from build123d import *

# Parameters (mm, degrees)
F0_W     = 76.2
F0_H     = 50.8
F0_R     = 12.7
F1_DEPTH = 12.7
F2_W     = 1.27
F2_H     = 50.8
F3_DEPTH = 5.08
F5_DEPTH = 50.801
F6_R     = 4.7625
F7_DEPTH = 12.7
F8_W     = 12.7
F8_H     = 50.8
F9_DEPTH = 6.35


with BuildPart() as f1:
    # F0 (on Top) → F1 (new body)
    with BuildSketch(Plane.XY):
        Rectangle(F0_W, F0_H)
        Circle(F0_R, mode=Mode.SUBTRACT)
    extrude(amount=-F1_DEPTH)

    # F2 (on face) → F3 (cut)
    with BuildSketch(Plane.XY):
        with Locations((-27.305, 0)):
            Rectangle(F2_W, F2_H)
        with BuildLine():
            Line((-6.35, -10.9985226281), (-6.35, -25.4))
            Line((-6.35, -25.4), (6.35, -25.4))
            Line((6.35, -25.4), (6.35, -10.9985226281))
            ThreePointArc((6.35, -10.9985226281), (0, -12.7), (-6.35, -10.9985226281))
        make_face()
        with BuildLine():
            Line((6.35, 25.4), (-6.35, 25.4))
            Line((-6.35, 25.4), (-6.35, 10.9985226281))
            ThreePointArc((-6.35, 10.9985226281), (0, 12.7), (6.35, 10.9985226281))
            Line((6.35, 10.9985226281), (6.35, 25.4))
        make_face()
    extrude(amount=-F3_DEPTH, mode=Mode.SUBTRACT)

    # F4 (on face) → F5 (cut, through all)
    with BuildSketch(Plane.XZ.offset(25.4)):
        Polygon((31.75, 0), (19.05, 0), (16.1170606325, -5.08), (34.6829393675, -5.08), align=None)
    extrude(amount=-F5_DEPTH, mode=Mode.SUBTRACT)

    # F6 (on face) → F7 (join)
    with BuildSketch(Plane.YZ.offset(38.1)):
        with Locations((0, -6.35)):
            Circle(F6_R)
    extrude(amount=F7_DEPTH)

    # F8 (on face) → F9 (join)
    with BuildSketch(Plane(origin=(0, 0, -12.7), x_dir=(1, 0, 0), z_dir=(0, 0, -1))):
        with Locations((-21.59, 0)):
            Rectangle(F8_W, F8_H)
        with Locations((21.59, 0)):
            Rectangle(F8_W, F8_H)
    extrude(amount=F9_DEPTH)


solid = f1.part
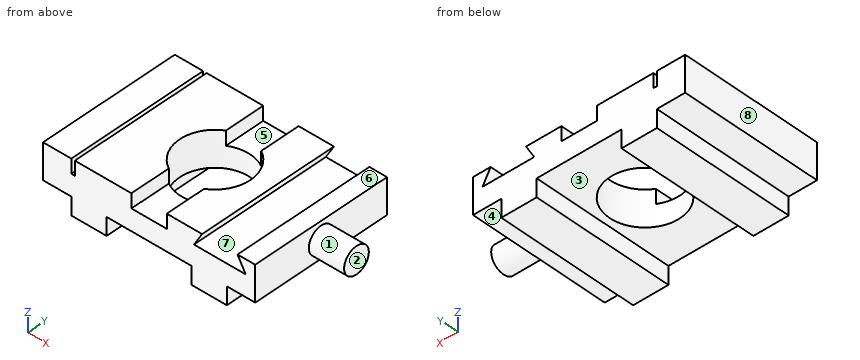
CAD build for the part. Positions are in the model's coordinates, mm. Face numbers are marked on the shaded views. A direction names the side the tool comes from. Coordinates: 2 decimals unless noted, no trailing zeros. Write each loop counter-clockwise with the first axis right and the second up, starting at its lowest first coordinate (ties: lowest second). Pieces come first, ordered by that corner, then holes. Notation, with made-up numbers: (12.25, -39.75) - (52.25, -39.75) arc R27 ccw to (52.25, -10.75) - close; hole circle Ø1 at (-24.5, 74.5). An arc over 180 degrees is marked (long way). Use a Markdown table: item, result. Add a question column.
Item 1: 3-axis set-ups, long thin cutter, end or side, ignore diameter. For the marked faces 1, 2, 3, 4 and 5: which of +Z, -Z, +X, -X, +Y, -Y reach the whole face in a straight line?
Item 2: Band-saw the part on B-B, the plane x = 0. Give the cut face in (y, z).
Item 3: Drill centre lines: L1, parallel to Y at x = 0, z = -5.75; L2, parallel to X at y = 10, z = -16; L3, parallel to X at y = 0, z = -6. Where is each one in solid material? Low to high. Write a range as from..to.
Item 4: Mould opens along Z. For the marked faces 6, 7 and 8 say: pulls with the +Z half, pulls with the -Z half, needs draft (parallel to the pull), parting line crosses it, or undercut.
Item 5: Band-saw the part on A-A, the plane y = 0. Give the cut face in (x, z).
Item 6: Band-saw the part on D-D, the plane y = 22. Give the cut face in (x, z), and give its area (3 significant figures).
Item 7: Flat gauge pins, fed straight in: pin 1 (1.5 mm diameter, centred on y = 19.5, z = -1.5, fed in from +X); pin 2 (4 mm diameter, centred on x = 2.5, y = -16, fed in from +Z); pin 3 (1.9 mm diameter, centred on y = 2, z = -15, fed in from +X); pin 4 (20.5 mm diameter, centred on x = 24, y = -5.5, fed in from +Z). Where does each tip first touch, or does it go through?
Item 8: Band-saw the part on C-C, the plane z = -6.35. Give the cut face in (x, y), and give its area (3 significant figures).
Numbers:
| question | item | result |
|---|---|---|
| 1 | face 1 | +X |
| 1 | face 2 | +Z, -Z, +X, +Y, -Y |
| 1 | face 3 | -Z, +Y, -Y |
| 1 | face 4 | -Z, +X, +Y, -Y |
| 1 | face 5 | +Z, +Y, -Y |
| 2 | outline | (-25.4, -12.7) - (-12.7, -12.7) - (-12.7, -5.08) - (-25.4, -5.08) - close; (12.7, -12.7) - (25.4, -12.7) - (25.4, -5.08) - (12.7, -5.08) - close |
| 3 | L1 | -25.4..-12.7, 12.7..25.4 |
| 3 | L2 | -27.94..-15.24, 15.24..27.94 |
| 3 | L3 | -38.1..-12.7, 12.7..50.8 |
| 4 | face 6 | pulls with the +Z half |
| 4 | face 7 | undercut |
| 4 | face 8 | needs draft |
| 5 | outline | (-38.1, -12.7) - (-27.94, -12.7) - (-27.94, -19.05) - (-15.24, -19.05) - (-15.24, -12.7) - (-12.7, -12.7) - (-12.7, 0) - (-26.67, 0) - (-26.67, -5.08) - (-27.94, -5.08) - (-27.94, 0) - (-38.1, 0) - close; (12.7, -12.7) - (15.24, -12.7) - (15.24, -19.05) - (27.94, -19.05) - (27.94, -12.7) - (38.1, -12.7) - (38.1, -11.11) - (50.8, -11.11) - (50.8, -1.59) - (38.1, -1.59) - (38.1, 0) - (31.75, 0) - (34.68, -5.08) - (16.12, -5.08) - (19.05, 0) - (12.7, 0) - close |
| 6 | outline | (-38.1, -12.7) - (-27.94, -12.7) - (-27.94, -19.05) - (-15.24, -19.05) - (-15.24, -12.7) - (15.24, -12.7) - (15.24, -19.05) - (27.94, -19.05) - (27.94, -12.7) - (38.1, -12.7) - (38.1, 0) - (31.75, 0) - (34.68, -5.08) - (16.12, -5.08) - (19.05, 0) - (6.35, 0) - (6.35, -5.08) - (-6.35, -5.08) - (-6.35, 0) - (-26.67, 0) - (-26.67, -5.08) - (-27.94, -5.08) - (-27.94, 0) - (-38.1, 0) - close |
| 6 | area | 979 mm2 |
| 7 | pin 1 | x = 38.1 |
| 7 | pin 2 | z = -5.08 |
| 7 | pin 3 | x = 27.94 |
| 7 | pin 4 | z = 0 |
| 8 | outline | (-38.1, -25.4) - (38.1, -25.4) - (38.1, -4.76) - (50.8, -4.76) - (50.8, 4.76) - (38.1, 4.76) - (38.1, 25.4) - (-38.1, 25.4) - close; hole circle Ø25.4 at (0, 0) |
| 8 | area | 3,490 mm2 |
